For this review, take the finished solid that the model builds, in its own axes (mm). Face numbers are marked on the shaded views. A direction names the side the tool comes from. Round coordinates to 2 decimals unless told otherwise and drop trailing zeros. Write each loop counter-clockwise with the first axis right and the second up, starting at its lowest first coordinate (ties: lowest second). Pieces come first, ordered by that corner, then holes. Notation, with made-up numbers: (-11, -15) -> (24, -15) arc R20 cw to (24, 3) -> close; hole circle Ø10 at (65, 18.5). An arc over 180 degrees is marked (long way). Answer in a Markdown table with one row per item. Add a question column.
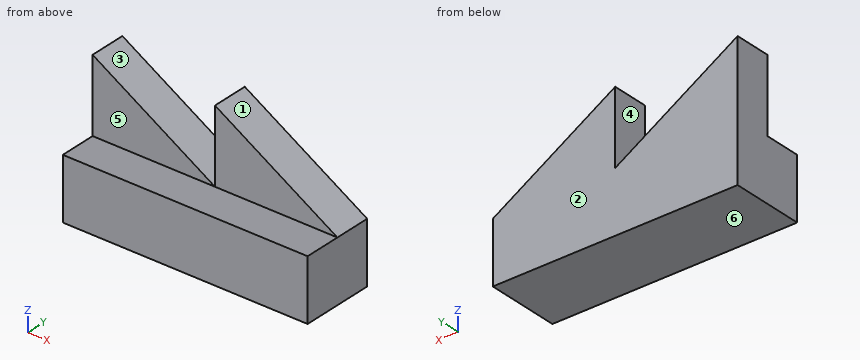
```python
from build123d import *

# Parameters (mm, degrees)
F1_DEPTH = 38.1
F2_DEPTH = 19.05


with BuildPart() as f1:
    # F0 (on Front) → F1 (new body)
    with BuildSketch(Plane.XZ):
        Polygon((-63.5, 0), (-63.5, -31.75), (63.5, -31.75), (63.5, 0), (0, 0), align=None)
    extrude(amount=F1_DEPTH)

    # F0 (on Front) → F2 (join)
    with BuildSketch(Plane.XZ):
        Polygon((-63.5, 38.1), (-63.5, 0), (0, 0), align=None)
        Polygon((0, 0), (63.5, 0), (0, 38.1), align=None)
    extrude(amount=F2_DEPTH)


solid = f1.part
```
1. Tool access review of the marked faces 4, 5 and 6: name each direction out of +Z, -Z, +X, -X, +Y, -Y from which nothing blocks a thin tool from reaching the whole face with its end or side.
2. The part is to be moulded in two halves that separate along X. For the marked faces 1, 2 and 3, say which applies: pulls with the +X half, pulls with the -X half, needs draft (parallel to the pull), parting line crosses it, or undercut.
3. We need section C-C (y = -15). Write out the cut boundary in (x, z), plus the area to 3 significant figures.
4. We need section D-D (z = 23). Write out the cut boundary in (x, y).
5. We need section A-A (z = 3.5). Write out the cut boundary in (x, y).
6. We need section B-B (x = 35.5). Write out the cut boundary in (y, z).
7. For L1, parallel to Z at x = -13, y = -27; L2, parallel to X at y = -15, z = 12.5; L3, parallel to X at y = -7, z = 25, list the stretches that pass through material, from the lowest coordinate up. Write a range as [from, to].
8. Clearance check with flat-ended pins moving along their axes: pin 1 Ø1.5 at (x, y) = (26, -32.5) entering from +Z; pin 2 Ø11.5 at (x, z) = (26, 15) entering from -Y; pin 3 Ø4 at (x, y) = (-9, -13.5) entering from +Z. State where each tip first meets the part, or that it passes through.
Response:
| question | item | result |
|---|---|---|
| 1 | face 4 | +Z, +Y, -Y |
| 1 | face 5 | +Z, +X, -X, -Y |
| 1 | face 6 | -Z, +X, -X, +Y, -Y |
| 2 | face 1 | pulls with the +X half |
| 2 | face 2 | needs draft |
| 2 | face 3 | undercut |
| 3 | outline | (-63.5, -31.75) -> (63.5, -31.75) -> (63.5, 0) -> (0, 38.1) -> (0, 0) -> (-63.5, 38.1) -> close |
| 3 | area | 6,450 mm2 |
| 4 | outline | (-63.5, -19.05) -> (-38.33, -19.05) -> (-38.33, 0) -> (-63.5, 0) -> close; (0, -19.05) -> (25.17, -19.05) -> (25.17, 0) -> (0, 0) -> close |
| 5 | outline | (-63.5, -19.05) -> (-5.83, -19.05) -> (-5.83, 0) -> (-63.5, 0) -> close; (0, -19.05) -> (57.67, -19.05) -> (57.67, 0) -> (0, 0) -> close |
| 6 | outline | (-38.1, -31.75) -> (0, -31.75) -> (0, 16.8) -> (-19.05, 16.8) -> (-19.05, 0) -> (-38.1, 0) -> close |
| 7 | L1 | [-31.75, 0] |
| 7 | L2 | [-63.5, -20.83], [0, 42.67] |
| 7 | L3 | [-63.5, -41.67], [0, 21.83] |
| 8 | pin 1 | z = 0 |
| 8 | pin 2 | y = -19.05 |
| 8 | pin 3 | z = 6.6 |
